For this review, use the dimensioned drawing (mm, ordinates from the lowest corner) and the shaded views. A direction names the side the tool comes from. Round coordinates to 2 decimals unless told otherwise and drop trailing zeros. Order: outer loops, then holes, each group sorted by start corner. A loop starts at its lowest first (then second) coordinate and runs counter-clockwise, first axis right, second up. Notation, with made-up numbers: M 48,2.25 L 92,2.25 A27 ccw 92,26.25 Z; hole C -5,-29.5 d4. An arc over 180 degrees is marked long. Put each result on its own line as item: value.
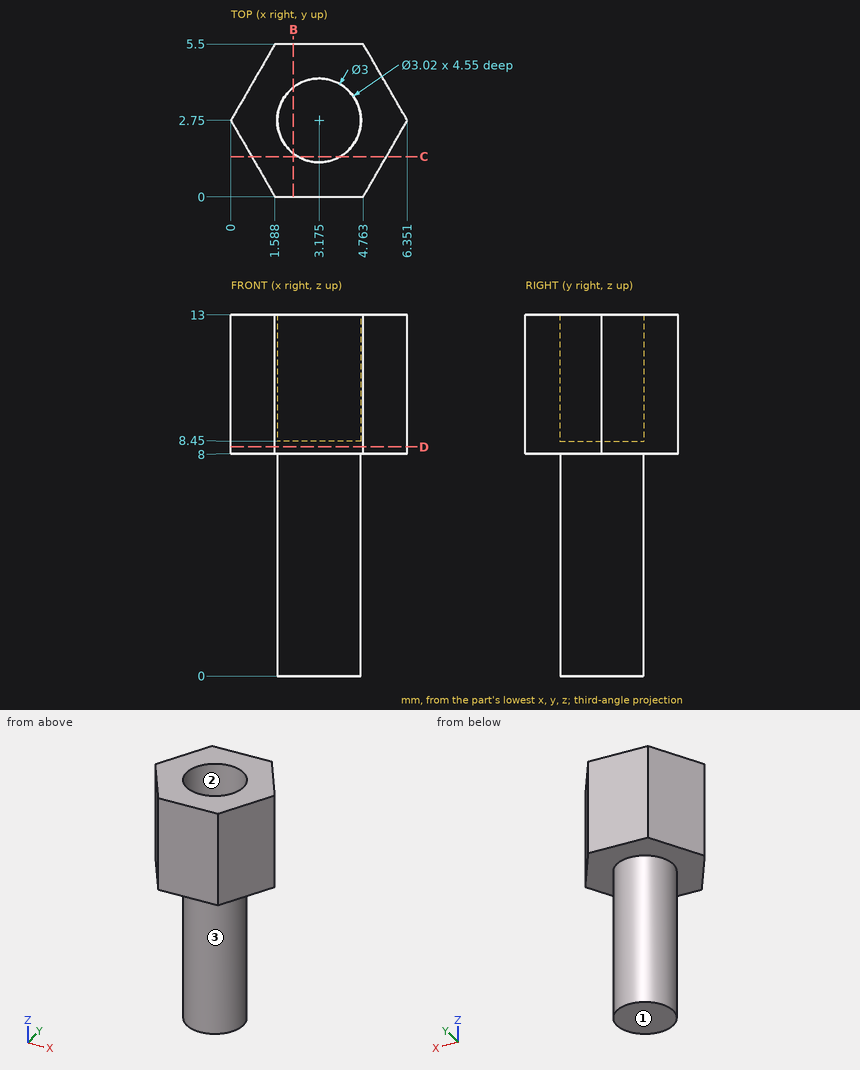
(1) Add section C-C on y = 1.45. Give the boundary of the cut face in (x, z).
A:
outline: M 0.75,8 L 2.43,8 L 2.43,0 L 3.92,0 L 3.92,8 L 5.6,8 L 5.6,13 L 3.94,13 L 3.94,8.45 L 2.41,8.45 L 2.41,13 L 0.75,13 Z
(2) Insertion check: pin 1 Ø1 at (y, z) = (4, 8.5) entering from +X; pin 2 Ø2 at (y, z) = (3, 2.5) entering from -X (1 decimal); pin 3 Ø1 at (y, z) = (1, 9.5) entering from +X. Each pin has a flat end and moves straight along its axis. Give the tip position at first contact, or say it passes through.
A:
pin 1: stops at x = 5.92
pin 2: stops at x = 1.7
pin 3: stops at x = 5.63
(3) To check wall thickness, follow L1, parallel to Z at x = 2.75, y = 3.2; L2, parallel to Z at x = 2.75, y = 4.95; L3, parallel to X at y = 3, z = 10.5 (1 decimal). State the ranges of each line that lie inside material, in increasing order.
A:
L1: z = 0 to 8.45
L2: z = 8 to 13
L3: x = 0.1 to 1.7, 4.7 to 6.2
(4) Add section D-D on z = 8.25. Give the boundary of the cut face in (x, y).
A:
outline: M 0,2.75 L 1.59,0 L 4.76,0 L 6.35,2.75 L 4.76,5.5 L 1.59,5.5 Z
(5) Add section B-B on x = 2.25. Give the boundary of the cut face in (y, z).
A:
outline: M 0,8 L 1.57,8 L 1.57,0 L 3.93,0 L 3.93,8 L 5.5,8 L 5.5,13 L 3.94,13 L 3.94,8.45 L 1.56,8.45 L 1.56,13 L 0,13 Z
(6) For the marked faces 1, 2 and 3, list the 3-axis set-ups (+Z, -Z, +X, -X, +Y, -Y) from which the entire face can be reached by the end or side of a thin tool; tool diameter is ignored.
A:
face 1: -Z, +X, -X, +Y, -Y
face 2: +Z
face 3: -Z
